```python
from build123d import *

# Parameters (mm, degrees)
F0_R     = 1
F1_DEPTH = 1.5
F2_R     = 5
F3_DEPTH = 10
F5_DEPTH = 10
F7_D     = 2.5


with BuildPart() as f1:
    # F0 (on Right) → F1 (new body)
    with BuildSketch(Plane.YZ):
        Polygon((0, 78), (0, 0), (32, 0), (32, 78), (20, 78), (20, 75.5), (12, 75.5), (12, 78), align=None)
        with Locations((3, 32)):
            Circle(F0_R, mode=Mode.SUBTRACT)
        with Locations((29, 32)):
            Circle(F0_R, mode=Mode.SUBTRACT)
    extrude(amount=F1_DEPTH)

    # F2 (on face) → F3 (join)
    with BuildSketch(Plane.YZ.offset(1.5)):
        with Locations((16, 25)):
            Circle(F2_R)
    extrude(amount=F3_DEPTH)

    # F4 (on face) → F5 (join)
    with BuildSketch(Plane.YZ.offset(1.5)):
        Polygon((20, 70), (16, 70), (12, 70), (12, 62), (20, 62), align=None)
    extrude(amount=F5_DEPTH)

    # F7 (through all)
    with Locations(Plane.YZ.offset(1.5)):
        with Locations((5, 73), (27, 73), (27, 5), (8, 5)):
            Hole(F7_D / 2)


solid = f1.part
```
The model under review builds one solid part; all positions refer to its coordinate system, in mm. A direction names the side the tool comes from. Give positions to 0.01 mm unless a question says otherwise; leave off trailing zeros. Write each loop counter-clockwise with the first axis right and the second up, starting at its lowest first coordinate (ties: lowest second). Pieces come first, ordered by that corner, then holes.
(1) The part is to be moulded in two halves that separate along Y. For faces 5 (the flat face through (1, 0, 40)), 6 (the flat face through (1, 32, 38)), 7 (the cylindrical face through (0.74, 25.845, 4.521)), 8 (the cylindrical face through (0.74, 5.16, 74.24)), say which applies: released by +Y, released by -Y, zero draft, split by the parting line, or undercut.
(2) Consider section A-A, the plane z = 73. Give the boundary of the cut face in (x, y).
(3) Consider section B-B, the plane y = 8. Give the boundary of the cut face in (x, z), and give its area (3 significant figures).
(4) To check wall thickness, follow L1, parallel to Z at x = 0.65, y = 27; L2, parallel to Y at x = 1.1, z = 73; L3, parallel to X at y = 5.5, z = 20. State the ranges of each line that lie inside material, in increasing order.
(5) For P1, Ø4, axis at x = 4.5, z = 68, coming from the -Y side; P2, Ø4, axis at x = 8, y = 18, coming from the -Z side; P3, Ø12, axis at y = 3.5, z = 60.5, coming from the +X side; P4, Ø5, axis at y = 13, z = 56.5, coming from the -X side, all flat-tipped, find the tip position at first contact; note any pin that passes through.
(6) Consider section C-C, the plane y = 16. Give the boundary of the cut face in (x, z), and give its area (3 significant figures).
(7) Tool access review of faces 1 (the flat face through (6, 16, 70)), 2 (the flat face through (6, 16, 62)), 3 (the cylindrical face through (6.43, 18.307, 20.564)), 4 (the flat face through (6, 20, 66)): name each direction out of +Z, -Z, +X, -X, +Y, -Y from which nothing blocks a thin tool from reaching the whole face with its end or side.
(8) Consider section D-D, the plane z = 25. Give the boundary of the cut face in (x, y), and give its area (3 significant figures).
Returned:
1. face 5: released by -Y
1. face 6: released by +Y
1. face 7: undercut
1. face 8: undercut
2. outline: (0, 0) - (1.5, 0) - (1.5, 3.75) - (0, 3.75) - close; (0, 6.25) - (1.5, 6.25) - (1.5, 25.75) - (0, 25.75) - close; (0, 28.25) - (1.5, 28.25) - (1.5, 32) - (0, 32) - close
3. outline: (0, 0) - (1.5, 0) - (1.5, 3.75) - (0, 3.75) - close; (0, 6.25) - (1.5, 6.25) - (1.5, 78) - (0, 78) - close
3. area: 113 mm2
4. L1: z = 0 to 3.75, 6.25 to 71.75, 74.25 to 78
4. L2: y = 0 to 3.75, 6.25 to 25.75, 28.25 to 32
4. L3: x = 0 to 1.5
5. P1: stops at y = 12
5. P2: stops at z = 20
5. P3: stops at x = 1.5
5. P4: stops at x = 0
6. outline: (0, 0) - (1.5, 0) - (1.5, 20) - (11.5, 20) - (11.5, 30) - (1.5, 30) - (1.5, 62) - (11.5, 62) - (11.5, 70) - (1.5, 70) - (1.5, 75.5) - (0, 75.5) - close
6. area: 293 mm2
7. face 1: +Z, +X, +Y, -Y
7. face 2: +X, +Y, -Y
7. face 3: +X
7. face 4: +Z, +X, +Y
8. outline: (0, 0) - (1.5, 0) - (1.5, 11) - (11.5, 11) - (11.5, 21) - (1.5, 21) - (1.5, 32) - (0, 32) - close
8. area: 148 mm2
